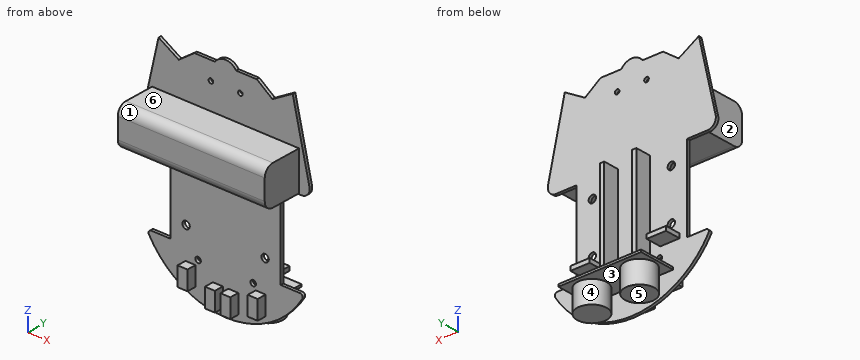
```python
from build123d import *

# Parameters (mm, degrees)
BOSS_EXTRUDE1_DEPTH = 1.6
SKETCH6_W           = 45
SKETCH6_H           = 1.2
BOSS_EXTRUDE2_DEPTH = 20
SKETCH7_R           = 8
BOSS_EXTRUDE3_DEPTH = 12
SKETCH10_W          = 80
SKETCH10_H          = 21
BOSS_EXTRUDE4_DEPTH = 21.4
FILLET1_R           = 5
CUT_EXTRUDE1_REACH  = 132.929
SKETCH11_R          = 1.25
SKETCH11_R_2        = 2
SKETCH11_R_3        = 1.5
SKETCH12_W          = 2.3
SKETCH12_H          = 51
SKETCH12_W_2        = 10.5
SKETCH12_H_2        = 2.3
BOSS_EXTRUDE5_DEPTH = 8.5
SKETCH13_W          = 5.4
SKETCH13_H          = 10.2
BOSS_EXTRUDE7_DEPTH = 5


with BuildPart() as part:
    # Sketch5 → Boss-Extrude1 (new body)
    with BuildSketch(Plane(origin=(0, 0, 0), x_dir=(1, 0, 0), z_dir=(0, 1, 0))):
        with BuildLine():
            Line((-25.5, 9.227208522), (-17, 3))
            Line((-17, 3), (-5.744562647, 3))
            ThreePointArc((-5.744562647, 3), (0, 0), (5.744562647, 3))
            Line((5.744562647, 3), (17, 3))
            Line((17, 3), (25.5, 9.227208522))
            Line((25.5, 9.227208522), (36.5, 2.727208522))
            Line((36.5, 2.727208522), (45.638339075, 42.980975538))
            ThreePointArc((45.638339075, 42.980975538), (44.766606918, 46.784961322), (41.25, 48.477208522))
            Line((41.25, 48.477208522), (30, 48.477208522))
            Line((30, 48.477208522), (30, 94.477208522))
            Line((30, 94.477208522), (40.42392202, 94.477208522))
            ThreePointArc((40.42392202, 94.477208522), (41.72734925, 95.234862609), (41.714047191, 96.742438582))
            ThreePointArc((41.714047191, 96.742438582), (0, 120.5), (-41.714047191, 96.742438582))
            ThreePointArc((-41.714047191, 96.742438582), (-41.72734925, 95.234862609), (-40.42392202, 94.477208522))
            Line((-40.42392202, 94.477208522), (-30, 94.477208522))
            Line((-30, 94.477208522), (-30, 48.477208522))
            Line((-30, 48.477208522), (-41.25, 48.477208522))
            ThreePointArc((-41.25, 48.477208522), (-44.766606918, 46.784961322), (-45.638339075, 42.980975538))
            Line((-45.638339075, 42.980975538), (-36.5, 2.727208522))
            Line((-36.5, 2.727208522), (-25.5, 9.227208522))
        make_face()
    extrude(amount=-BOSS_EXTRUDE1_DEPTH)

    # Sketch6 → Boss-Extrude2 (add)
    with BuildSketch(Plane(origin=(0, 0, 0), x_dir=(1, 0, 0), z_dir=(0, 1, 0))):
        with Locations((0, 106.3)):
            Rectangle(SKETCH6_W, SKETCH6_H)
    extrude(amount=BOSS_EXTRUDE2_DEPTH)

    # Sketch7 → Boss-Extrude3 (add)
    with BuildSketch(Plane(origin=(0, 0, -106.9), x_dir=(-1, 0, 0), z_dir=(0, 0, -1))):
        with Locations(Location((-13, 10, 0), (0, 0, 180))):
            Circle(SKETCH7_R)
        with Locations(Location((13, 10, 0), (0, 0, 180))):
            Circle(SKETCH7_R)
    extrude(amount=BOSS_EXTRUDE3_DEPTH)

    # Sketch10 → Boss-Extrude4 (add)
    with BuildSketch(Plane.XZ.offset(1.6)):
        with Locations((0, -37.5)):
            Rectangle(SKETCH10_W, SKETCH10_H)
    extrude(amount=BOSS_EXTRUDE4_DEPTH)

    # Fillet1
    fillet1_edges = [part.edges().sort_by_distance(p)[0] for p in [
        (0, -23, -48),
        (0, -23, -27),
    ]]
    fillet(fillet1_edges, radius=FILLET1_R)

    # Sketch11 → Cut-Extrude1 (cut, up to next)
    with BuildSketch(Plane(origin=(0, 0, 0), x_dir=(1, 0, 0), z_dir=(0, 1, 0)), mode=Mode.PRIVATE) as cut_extrude1_sk1:
        with Locations(Location((-8, 12.8, 0), (0, 0, 270))):
            Circle(SKETCH11_R)
    cut_extrude1_tool1 = extrude(cut_extrude1_sk1.sketch, amount=-CUT_EXTRUDE1_REACH, mode=Mode.PRIVATE) & part.part
    # Sketch11 → Cut-Extrude1 (cut, up to next)
    with BuildSketch(Plane(origin=(0, 0, 0), x_dir=(1, 0, 0), z_dir=(0, 1, 0)), mode=Mode.PRIVATE) as cut_extrude1_sk2:
        with Locations(Location((-21.5, 58, 0), (0, 0, 270))):
            Circle(SKETCH11_R_2)
    cut_extrude1_tool2 = extrude(cut_extrude1_sk2.sketch, amount=-CUT_EXTRUDE1_REACH, mode=Mode.PRIVATE) & part.part
    # Sketch11 → Cut-Extrude1 (cut, up to next)
    with BuildSketch(Plane(origin=(0, 0, 0), x_dir=(1, 0, 0), z_dir=(0, 1, 0)), mode=Mode.PRIVATE) as cut_extrude1_sk3:
        with Locations(Location((-21.5, 85, 0), (0, 0, 270))):
            Circle(SKETCH11_R_2)
    cut_extrude1_tool3 = extrude(cut_extrude1_sk3.sketch, amount=-CUT_EXTRUDE1_REACH, mode=Mode.PRIVATE) & part.part
    # Sketch11 → Cut-Extrude1 (cut, up to next)
    with BuildSketch(Plane(origin=(0, 0, 0), x_dir=(1, 0, 0), z_dir=(0, 1, 0)), mode=Mode.PRIVATE) as cut_extrude1_sk4:
        with Locations(Location((-15, 99, 0), (0, 0, 270))):
            Circle(SKETCH11_R_3)
    cut_extrude1_tool4 = extrude(cut_extrude1_sk4.sketch, amount=-CUT_EXTRUDE1_REACH, mode=Mode.PRIVATE) & part.part
    # Sketch11 → Cut-Extrude1 (cut, up to next)
    with BuildSketch(Plane(origin=(0, 0, 0), x_dir=(1, 0, 0), z_dir=(0, 1, 0)), mode=Mode.PRIVATE) as cut_extrude1_sk5:
        with Locations(Location((15, 99, 0), (0, 0, 90))):
            Circle(SKETCH11_R_3)
    cut_extrude1_tool5 = extrude(cut_extrude1_sk5.sketch, amount=-CUT_EXTRUDE1_REACH, mode=Mode.PRIVATE) & part.part
    # Sketch11 → Cut-Extrude1 (cut, up to next)
    with BuildSketch(Plane(origin=(0, 0, 0), x_dir=(1, 0, 0), z_dir=(0, 1, 0)), mode=Mode.PRIVATE) as cut_extrude1_sk6:
        with Locations(Location((21.5, 85, 0), (0, 0, 90))):
            Circle(SKETCH11_R_2)
    cut_extrude1_tool6 = extrude(cut_extrude1_sk6.sketch, amount=-CUT_EXTRUDE1_REACH, mode=Mode.PRIVATE) & part.part
    # Sketch11 → Cut-Extrude1 (cut, up to next)
    with BuildSketch(Plane(origin=(0, 0, 0), x_dir=(1, 0, 0), z_dir=(0, 1, 0)), mode=Mode.PRIVATE) as cut_extrude1_sk7:
        with Locations(Location((21.5, 58, 0), (0, 0, 90))):
            Circle(SKETCH11_R_2)
    cut_extrude1_tool7 = extrude(cut_extrude1_sk7.sketch, amount=-CUT_EXTRUDE1_REACH, mode=Mode.PRIVATE) & part.part
    # Sketch11 → Cut-Extrude1 (cut, up to next)
    with BuildSketch(Plane(origin=(0, 0, 0), x_dir=(1, 0, 0), z_dir=(0, 1, 0)), mode=Mode.PRIVATE) as cut_extrude1_sk8:
        with Locations(Location((8, 12.8, 0), (0, 0, 90))):
            Circle(SKETCH11_R)
    cut_extrude1_tool8 = extrude(cut_extrude1_sk8.sketch, amount=-CUT_EXTRUDE1_REACH, mode=Mode.PRIVATE) & part.part
    add(cut_extrude1_tool1.solids().sort_by_distance((-8, 0, -12.8))[0], mode=Mode.SUBTRACT)
    add(cut_extrude1_tool2.solids().sort_by_distance((-21.5, 0, -58))[0], mode=Mode.SUBTRACT)
    add(cut_extrude1_tool3.solids().sort_by_distance((-21.5, 0, -85))[0], mode=Mode.SUBTRACT)
    add(cut_extrude1_tool4.solids().sort_by_distance((-15, 0, -99))[0], mode=Mode.SUBTRACT)
    add(cut_extrude1_tool5.solids().sort_by_distance((15, 0, -99))[0], mode=Mode.SUBTRACT)
    add(cut_extrude1_tool6.solids().sort_by_distance((21.5, 0, -85))[0], mode=Mode.SUBTRACT)
    add(cut_extrude1_tool7.solids().sort_by_distance((21.5, 0, -58))[0], mode=Mode.SUBTRACT)
    add(cut_extrude1_tool8.solids().sort_by_distance((8, 0, -12.8))[0], mode=Mode.SUBTRACT)

    # Sketch12 → Boss-Extrude5 (add)
    with BuildSketch(Plane(origin=(0, 0, 0), x_dir=(1, 0, 0), z_dir=(0, 1, 0))):
        with Locations((-8.75, 74.5)):
            Rectangle(SKETCH12_W, SKETCH12_H)
        with Locations((-20.75, 92.35)):
            Rectangle(SKETCH12_W_2, SKETCH12_H_2)
        with Locations((20.75, 92.35)):
            Rectangle(SKETCH12_W_2, SKETCH12_H_2)
        with Locations((8.75, 74.5)):
            Rectangle(SKETCH12_W, SKETCH12_H)
    extrude(amount=BOSS_EXTRUDE5_DEPTH)

    # Sketch13 → Boss-Extrude7 (add)
    with BuildSketch(Plane.XZ.offset(1.6)):
        with Locations((4.2, -111.6)):
            Rectangle(SKETCH13_W, SKETCH13_H)
        with Locations((-4.2, -111.6)):
            Rectangle(SKETCH13_W, SKETCH13_H)
        with Locations((-19.1, -107)):
            Rectangle(SKETCH13_W, SKETCH13_H)
        with Locations((19.1, -107)):
            Rectangle(SKETCH13_W, SKETCH13_H)
    extrude(amount=BOSS_EXTRUDE7_DEPTH)


solid = part.part
```
Read the model definition and answer for the solid it produces. Units are mm, in the model's axes. Face numbers are marked on the shaded views. A direction names the side the tool comes from. Give positions to 0.01 mm unless a question says otherwise; leave off trailing zeros. Order: outer loops, then holes, each group sorted by start corner. A loop starts at its lowest first (then second) coordinate and runs counter-clockwise, first axis right, second up. Notation, with made-up numbers: (3, 88) -> (23, 88) arc R23 cw to (23, 96) -> close; hole circle Ø6 at (-1.75, 19.5). An arc over 180 degrees is marked (long way). Write item = value, one per line.
1. A cutting plane is placed at C-C, the plane y = 10. Write down the section's boundary in (x, z).
Numbers:
outline = (-22.5, -106.9) -> (-21, -106.9) -> (-21, -118.9) -> (-5, -118.9) -> (-5, -106.9) -> (5, -106.9) -> (5, -118.9) -> (21, -118.9) -> (21, -106.9) -> (22.5, -106.9) -> (22.5, -105.7) -> (-22.5, -105.7) -> close
2. A cutting plane is placed at D-D, the plane z = -28.5. Write down the section's boundary in (x, y), and give its area (3 significant figures).
Numbers:
outline = (-42.35, -1.6) -> (-40, -1.6) -> (-40, -21.57) -> (40, -21.57) -> (40, -1.6) -> (42.35, -1.6) -> (42.35, 0) -> (-42.35, 0) -> close
area = 1,730 mm²
3. A cutting plane is placed at B-B, the plane x = -32. Write down the section's boundary in (y, z).
Numbers:
outline = (-23, -43) arc R5 ccw to (-18, -48) -> (-1.6, -48) -> (-1.6, -48.48) -> (0, -48.48) -> (0, -5.39) -> (-1.6, -5.39) -> (-1.6, -27) -> (-18, -27) arc R5 ccw to (-23, -32) -> close; (-1.6, -108.45) -> (0, -108.45) -> (0, -94.48) -> (-1.6, -94.48) -> close
4. Given pin 1 (6 mm diameter, centred on x = -23.5, y = 5, fed in from -Z); pin 2 (3 mm diameter, centred on x = -10, z = -96.5, fed in from +Y); pin 3 (5.5 mm diameter, centred on x = -20, y = -4.5, fed in from -Z); pin 4 (2 mm diameter, centred on x = 8, z = -12.8, fed in from -Y), each flat-ended and moving along its own axis, determine where each tip first touches the part or whether it passes through.
Numbers:
pin_1 = -106.9
pin_2 = 8.5
pin_3 = -112.1
pin_4 = through
5. For the marked faces 4, 5 and 6, determine the directions among +Z, -Z, +X, -X, +Y, -Y from which every point of the face is accessible in a straight line to the end or side of a thin tool.
Numbers:
face_4 = -Z
face_5 = -Z, +X, -X, +Y
face_6 = +Z, +X, -X, -Y
6. The mould has two halves that part along Y. Classify the marked faces 1, 2 and 3: +Y half, -Y half, draft (parallel to the pull), parting line (faces both ways), or undercut.
Numbers:
face_1 = -Y half
face_2 = draft
face_3 = undercut
7. Straight lines are drawn through the part: line 1 along Y through (x, z) = (13, -112); line 2 along X through (y, z) = (-0.6, -12.8); line 3 along X through (y, z) = (-1, -12). For each, find the intervals that lie inside material, in ascending order.
Numbers:
line_1 = -1.6 to 0, 2 to 18
line_2 = -38.79 to -9.25, -6.75 to 6.75, 9.25 to 38.79
line_3 = -38.61 to -8.96, -7.04 to 7.04, 8.96 to 38.61
8. A cutting plane is placed at A-A, the plane z = -58. Write down the section's boundary in (x, y).
Numbers:
outline = (-30, -1.6) -> (-23.5, -1.6) -> (-23.5, 0) -> (-30, 0) -> close; (-19.5, -1.6) -> (19.5, -1.6) -> (19.5, 0) -> (9.9, 0) -> (9.9, 8.5) -> (7.6, 8.5) -> (7.6, 0) -> (-7.6, 0) -> (-7.6, 8.5) -> (-9.9, 8.5) -> (-9.9, 0) -> (-19.5, 0) -> close; (23.5, -1.6) -> (30, -1.6) -> (30, 0) -> (23.5, 0) -> close
